Work out the finished part from the listing and answer in its coordinate system (mm). Round coordinates to 2 decimals unless told otherwise and drop trailing zeros. Order: outer loops, then holes, each group sorted by start corner. A loop starts at its lowest first (then second) coordinate and runs counter-clockwise, first axis right, second up. Notation, with made-up numbers: (39.5, 88.25) - (65.5, 88.25) arc R22 ccw to (65.5, 102.25) - close; hole circle Ø6 at (32.25, -18). An arc over 180 degrees is marked (long way). Put each result on its own line as item: value.
Autodesk Inventor part; units mm, degrees
ref_plane "YZ Plane" through (0, 0, 0) normal (1, 0, 0) x (0, 1, 0)
ref_plane "XZ Plane" through (0, 0, 0) normal (0, 1, 0) x (-1, 0, 0)
ref_plane "XY Plane" through (0, 0, 0) normal (0, 0, 1) x (1, 0, 0)
sketch "Sketch1" plane through (0, 0, 0) normal (0, 1, 0) x (-1, 0, 0)
  circle A0 centre (0, 0) radius 4
  dimension "d0" = 8
extrude "Extrusion1" add sketch "Sketch1" along normal blind 433.3875
sketch "Sketch2" plane through (0, 433.3875, 0) normal (0, 1, 0) x (1, 0, 0)
  circle A0 centre (0, 0) radius 4
  line L0 (6.5, -6.5) -> (-6.5, -6.5)
  line L1 (-6.5, -6.5) -> (-6.5, 6.5)
  line L2 (-6.5, 6.5) -> (6.5, 6.5)
  line L3 (6.5, 6.5) -> (6.5, -6.5)
  line L4 (6.5, -6.5) -> (-6.5, 6.5) construction
  line L5 (-6.5, -6.5) -> (6.5, 6.5) construction
  dimension "d3" = 13
  dimension "d4" = 13
extrude "Extrusion2" add sketch "Sketch2" along normal blind 41 contours A0 | L0 L1 L2 L3
sketch "Sketch3" plane through (-6.5, 433.3875, -6.5) normal (-1, 0, 0) x (0, 0, 1)
  line L0 (13, 0) -> (13, 41)
  line L1 (0, 0) -> (0, 41)
  line L2 (13, 41) -> (0, 41)
  arc A0 (15.4333, 39.9065) -> (-2.4333, 39.9065) centre (6.5, 41) ccw
  line L3 (13, 0) -> (15.5, 41)
  line L4 (0, 0) -> (-2.5, 41)
  point P0 (6.5, -433.3875)
  dimension "d7" = 18
extrude "Extrusion3" add sketch "Sketch3" against normal blind 13 contours L0 L2 L1 L4 A0 L3
sketch "Sketch4" plane through (-6.5, 474.3875, 0) normal (-1, 0, 0) x (0, 0, 1)
  arc A0 (9, 0) -> (-9, 0) centre (0, 0) ccw
  circle A1 centre (0, 0) radius 4.5
  point P0 (0, -474.3875)
  dimension "d11" = 9
extrude "Extrusion4" cut sketch "Sketch4" against normal blind 15
sketch "Sketch5" plane through (6.5, 433.3875, 6.5) normal (1, 0, 0) x (0, 0, -1)
  line L0 (13, 0) -> (15.5, 41)
  line L1 (13, 0) -> (14.2173, 19.9629)
  circle A0 centre (6.5, 41) radius 4.5
  line L2 (14.2173, 19.9629) -> (6.5, 41)
  line L3 (14.2173, 19.9629) -> (6.5, 41)
  line L4 (6.5, 41) -> (7.4388, 41.3444)
  line L5 (7.4388, 41.3444) -> (15.1561, 20.3073)
  line L6 (15.1561, 20.3073) -> (14.2173, 19.9629)
  point P0 (6.5, -433.3875)
  dimension "d25" = 20
  dimension "d26" = 1
extrude "Extrusion5" [suppressed]
sketch "Sketch6" plane through (6.5, 433.3875, -6.5) normal (0, -0.0609, -0.9981) x (-1, 0, 0)
  line L0 (13, 20) -> (0, 20)
  line L1 (13, 0) -> (0, 0)
  line L2 (6.5, 0) -> (6.5, 32)
  point P0 (6.5, -432.9797)
  dimension "d29" = 32
hole "Hole2" [suppressed]
thread "Thread2"
sketch "Sketch7" plane through (0, 0, 0) normal (1, 0, 0) x (0, 1, 0)
  line L0 (0, 0) -> (12.7, 0)
  line L1 (0, 0) -> (-16.3, 0)
  line L2 (0, 0) -> (-1.8, 0)
  arc A0 (-1.8, 14.5) -> (-1.8, -14.5) centre (-1.8, 0) ccw
  line L3 (-1.8, 14.5) -> (-1.8, -14.5)
  dimension "d41" = 12.7
  dimension "d43" = 1.8
revolve "Revolution1" cut sketch "Sketch7" angle 360 about axis through (0, -1.8, 14.5) along (0, 0, -1)
properties part number "Rod"
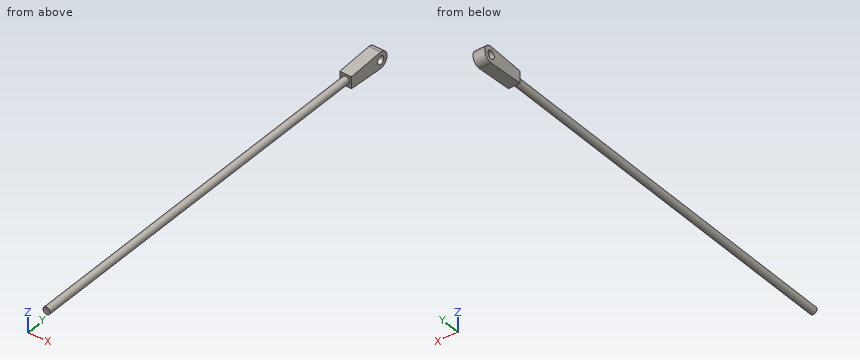
1) A cutting plane is placed at B-B on x = -1. Write down the section's boundary in (y, z), then the cut area to 3 significant figures.
Findings below:
outline: (12.14, -3.87) - (433.39, -3.87) - (433.39, -6.5) - (474.39, -9) arc R9 ccw to (474.39, 9) - (433.39, 6.5) - (433.39, 3.87) - (12.14, 3.87) arc R14.47 cw to start; hole circle Ø9 at (474.39, 0)
area: 3,960 mm2
2) Given pin 1 Ø4 at (x, z) = (-1.5, -2.5) entering from -Y; pin 2 Ø8 at (y, z) = (197, -6) entering from +X; pin 3 Ø4 at (x, y) = (3, 189.5) entering from -Z; pin 4 Ø3 at (x, y) = (-2, 195.5) entering from -Z, each flat-ended and moving along its own axis, determine where each tip first touches the part or whether it passes through.
Findings below:
pin 1: stops at y = 12.14
pin 2: stops at x = 3.46
pin 3: stops at z = -3.87
pin 4: stops at z = -3.97
3) Straight lines are drawn through the part: L1, parallel to Y at x = 5.5, z = -0.5; L2, parallel to Y at x = -0.75, z = 1.75; L3, parallel to X at y = 327, z = 1. For each, find the intervals that lie inside material, in ascending order. Write a range as from..to.
Findings below:
L1: y = 433.39..469.92, 478.86..483.37
L2: y = 12.57..470.24, 478.53..483.22
L3: x = -3.87..3.87
4) A cutting plane is placed at A-A on z = 0. Write down the section's boundary in (x, y).
Findings below:
outline: (-6.5, 433.39) - (-4, 433.39) - (-4, 12.14) arc R14.5 cw to (4, 12.14) - (4, 433.39) - (6.5, 433.39) - (6.5, 469.89) - (-6.5, 469.89) - close; (-6.5, 478.89) - (6.5, 478.89) - (6.5, 483.39) - (-6.5, 483.39) - close
5) A cutting plane is placed at C-C on y = 354.5. Write down the section's boundary in (x, z).
Findings below:
outline: circle Ø8 at (0, 0)
